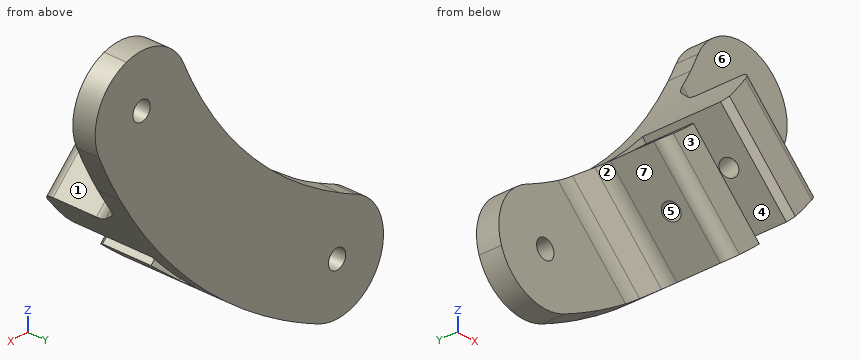
```python
from build123d import *

# Parameters (mm, degrees)
SKETCH1_R           = 1.7
BOSS_EXTRUDE1_DEPTH = 4
SKETCH2_W           = 8
SKETCH2_H           = 15
BOSS_EXTRUDE2_DEPTH = 30
CUT_EXTRUDE1_DEPTH  = 30
SKETCH4_R           = 1.5
CUT_EXTRUDE2_DEPTH  = 52.989471847
FILLET1_R           = 2
CHAMFER1_SIZE       = 1
CHAMFER2_SIZE       = 4
FILLET2_R           = 3


with BuildPart() as part:
    # Sketch1 → Boss-Extrude1 (new body)
    with BuildSketch(Plane.XZ.offset(74.901515315)):
        with BuildLine():
            ThreePointArc((21.566916187, -71.495231174), (26.53319413, -76.858714128), (33.842822155, -76.844426529))
            ThreePointArc((33.842822155, -76.844426529), (59.373405242, -59.373405242), (76.844426529, -33.842822155))
            ThreePointArc((76.844426529, -33.842822155), (76.858714128, -26.53319413), (71.495231174, -21.566916187))
            ThreePointArc((71.495231174, -21.566916187), (64.870172632, -21.821666174), (60.172932274, -26.500579645))
            ThreePointArc((60.172932274, -26.500579645), (46.492270863, -46.492270863), (26.500579645, -60.172932274))
            ThreePointArc((26.500579645, -60.172932274), (21.821666174, -64.870172632), (21.566916187, -71.495231174))
        make_face()
        with Locations((30.1717009, -68.508679402)):
            Circle(SKETCH1_R, mode=Mode.SUBTRACT)
        with Locations((68.508679402, -30.1717009)):
            Circle(SKETCH1_R, mode=Mode.SUBTRACT)
    extrude(amount=BOSS_EXTRUDE1_DEPTH)

    # Sketch2 → Boss-Extrude2 (add)
    with BuildSketch(Plane(origin=(62.280244247, 0, -62.280244247), x_dir=(-0.707106781, 0, -0.707106781), z_dir=(0.707106781, 0, -0.707106781))):
        with Locations((-8, -86.401515315)):
            Rectangle(SKETCH2_W, SKETCH2_H)
        Polygon((4, -93.901515315), (12, -93.901515315), (12, -78.901515315), (8, -78.901515315), (8, -81.901515315), (4, -84.210916392), align=None)
    extrude(amount=-BOSS_EXTRUDE2_DEPTH)

    # Sketch3 → Cut-Extrude1 (cut)
    with BuildSketch(Plane.XZ.offset(93.901515315)):
        with BuildLine():
            Line((29.484052126, -58.768641044), (22.062889108, -51.347478026))
            Line((22.062889108, -51.347478026), (52.677923164, -23.025448826))
            Line((52.677923164, -23.025448826), (58.652501829, -29.714416185))
            ThreePointArc((58.652501829, -29.714416185), (46.400970155, -46.583392627), (29.484052126, -58.768641044))
        make_face()
        with BuildLine():
            Line((72.712363398, -41.991840982), (86.447631041, -52.417601978))
            Line((86.447631041, -52.417601978), (48.404595932, -83.58162252))
            Line((48.404595932, -83.58162252), (40.796709535, -73.389583669))
            ThreePointArc((40.796709535, -73.389583669), (58.885753549, -59.857084201), (72.712363398, -41.991840982))
        make_face()
    extrude(amount=-CUT_EXTRUDE1_DEPTH, mode=Mode.SUBTRACT)

    # Sketch4 → Cut-Extrude2 (cut, through all)
    with BuildSketch(Plane(origin=(8.485281374, 0, 8.485281374), x_dir=(0.707106781, 0, -0.707106781), z_dir=(0.707106781, 0, 0.707106781))):
        with Locations((74.128214207, -88.901515315)):
            Circle(SKETCH4_R)
    extrude(amount=-CUT_EXTRUDE2_DEPTH, mode=Mode.SUBTRACT)

    # Fillet1
    fillet1_edges = [part.edges().sort_by_distance(p)[0] for p in [
        (43.752386609, -93.901515315, -60.722949357),
        (60.722949357, -93.901515315, -43.752386609),
    ]]
    fillet(fillet1_edges, radius=FILLET1_R)

    # Chamfer1
    chamfer1_edges = [part.edges().sort_by_distance(p)[0] for p in [
        (50.0276489, -93.901515315, -55.684503149),
        (55.684503149, -93.901515315, -50.0276489),
    ]]
    chamfer(chamfer1_edges, length=CHAMFER1_SIZE)

    # Chamfer2
    chamfer2_edges = [part.edges().sort_by_distance(p)[0] for p in [
        (60.722949357, -78.901515315, -43.752386609),
        (43.752386609, -78.901515315, -60.722949357),
    ]]
    chamfer(chamfer2_edges, length=CHAMFER2_SIZE)

    # Fillet2
    fillet2_edges = [part.edges().sort_by_distance(p)[0] for p in [
        (63.00381198, -78.901515315, -40.376394982),
        (60.722949357, -82.901515315, -43.752386609),
        (43.752386609, -82.901515315, -60.722949357),
        (40.376394982, -78.901515315, -63.00381198),
    ]]
    fillet(fillet2_edges, radius=FILLET2_R)


solid = part.part
```
CAD build for the part. Positions are in the model's coordinates, mm. Face numbers are marked on the shaded views. A direction names the side the tool comes from. Coordinates: 2 decimals unless noted, no trailing zeros. Order: outer loops, then holes, each group sorted by start corner. A loop starts at its lowest first (then second) coordinate and runs counter-clockwise, first axis right, second up. Notation, with made-up numbers: (53, 21.5) - (66, 21.5) arc R10 cw to (66, 31.5) - close; hole circle Ø8 at (84.25, 14). An arc over 180 degrees is marked (long way). Use a Markdown table: item, result. Add a question column.
(1) Saw through at B-B (x = 73.5). Give the cut face in (y, z), then the cut area to 3 significant figures.
(2) Pull direction X, two halves, no side cores. Call the marked faces 1, 2, 3 and 4: +X half, -X half, draft (parallel to the pull), parting line (faces both ways), or undercut.
(3) Drill centre lines: line 1 along Z through (x, y) = (51, -86.5); line 2 along Z through (x, y) = (50, -82.75); line 3 along Y through (x, z) = (71.5, -41.5). Where is each one in solid material? Low to high. Write a range as [from, to].
(4) Saw through at A-A (y = -85.75). Give the cut face in (x, z).
(5) Flat gauge pins, fed straight in: pin 1 (4 mm diameter, centred on x = 41.5, y = -89, fed in from -Z); pin 2 (2 mm diameter, centred on x = 62.5, y = -86.5, fed in from -Z); pin 3 (10 mm diameter, centred on x = 64.5, z = -30, fed in from -Y); pin 4 (2.5 mm diameter, centred on x = 30.17, z = -68.51, fed in from -Y). Where does each tip first touch, or does it go through?
(6) Which spindle directions (+Z, -Z, +X, -X, +Y, -Y) get a long thin tool onto all of the face, cutting with end or side? Do the marked faces 5, 6 and 7. Say none if no direction does.
Solved:
| question | item | result |
|---|---|---|
| 1 | outline | (-78.9, -40.6) - (-74.9, -40.6) - (-74.9, -22.55) - (-78.9, -22.55) - close |
| 1 | area | 72.2 mm² |
| 2 | face 1 | +X half |
| 2 | face 2 | -X half |
| 2 | face 3 | draft |
| 2 | face 4 | undercut |
| 3 | line 1 | z = [-66.7, -56.66], [-45.34, -41.5] |
| 3 | line 2 | z = [-67.46, -59.24], [-44.34, -42.7] |
| 3 | line 3 | y = [-78.9, -74.9] |
| 4 | outline | (37.23, -54.2) - (50.28, -67.25) arc R83.97 ccw to (56.48, -62.13) - (43.58, -49.23) arc R65.75 cw to start; (49.23, -43.58) - (62.13, -56.48) arc R83.97 ccw to (67.25, -50.28) - (54.2, -37.23) arc R65.75 cw to start |
| 5 | pin 1 | stops at z = -60.19 |
| 5 | pin 2 | stops at z = -56.48 |
| 5 | pin 3 | stops at y = -78.9 |
| 5 | pin 4 | passes through |
| 6 | face 5 | none |
| 6 | face 6 | +Z, +X, -Y |
| 6 | face 7 | -Z, -X, -Y |
